Input: part model. Units: mm. Frame: model coordinates. Coordinates: 2 decimals unless noted, no trailing zeros. Write each loop counter-clockwise with the first axis right and the second up, starting at its lowest first coordinate (ties: lowest second). Pieces come first, ordered by that corner, then holes. Notation, with made-up numbers: M -5,48.5 L 36,48.5 A19 cw 36,80.5 Z; hole C 78,78 d11. An arc over 180 degrees is marked long. Write each question's results on one line, items separated by ' | '. Start each with the question number.
1. Ray query, probe 1 along Y at (x, z) = (-6, 5.25); probe 2 along Y at (x, z) = (-11.5, 1); probe 3 along X at (y, z) = (4.5, -4.5). Return the intervals inside material, ascending.
2. Section query A-A, the plane x = -7.5. Output: boundary loops of the cut face in (y, z).
3. First-contact query: pin 1 (8 mm diameter, centred on x = -16, z = -3.5, fed in from +Y); pin 2 (2 mm diameter, centred on x = -9, y = -2.5, fed in from +Z); pin 3 (4 mm diameter, centred on x = -11.5, z = 3, fed in from +Y). Flat tips, straight axial feed; report the tip coordinate or a pass-through.
4. Section query B-B, the plane y = -3.75. Output: boundary loops of the cut face in (x, z).
```python
from build123d import *

# Parameters (mm, degrees)
CROQUIS_BASE_DEPTH             = 6.9937
LENTE_PPAL_1_REACH             = 29.176
LENTE_PPAL_1_DIRECTION_2_REACH = 29.176
LENTE_PPAL_2_DEPTH             = 28.175928622
LENTE_PPAL_2_DEPTH_BACK        = 28.175928622
CROQUIS9_3_OUTSIDE_W           = 30.065
CROQUIS9_3_OUTSIDE_H           = 25.937
LENTE_START                    = -6.9937
LENTE_FRONTAL_DEPTH            = 13.9874
LENTE_START_2                  = -6.993701
LENTE_TRASERA_DEPTH            = 13.987402


with BuildPart() as part:
    # Croquis1 → croquis base (new, symmetric)
    with BuildSketch(Plane.XY):
        with BuildLine():
            Line((-8.981845695, 12.608155172), (-23.035921146, 11.871612288))
            Line((-23.035921146, 11.871612288), (-23.035921146, 11.54013782))
            ThreePointArc((-23.035921146, 11.54013782), (-20.949684518, 9.582335705), (-18.945192114, 7.540918896))
            add(Edge.make_bspline(
                [(-18.945192114, 7.540918896), (-10.215008384, -3.697644103), (-2.846604825, -5.059081104)],
                knots=[0.497667241, 0.497667241, 0.497667241, 0.49955428, 0.49955428, 0.49955428], degree=2, weights=[1, 1, 1]))
            add(Edge.make_bspline(
                [(-2.846604825, -5.059081104), (-2.498165198, -4.87297933), (-2.177330418, -4.684462446)],
                knots=[0.498812075, 0.498812075, 0.498812075, 0.498911556, 0.498911556, 0.498911556], degree=2, weights=[1, 1, 1]))
            Line((-2.177330418, -4.684462446), (-2.177330418, 6.186438919))
            add(Edge.make_bspline(
                [(-2.177330418, 6.186438919), (-4.063319702, 8.141636997), (-6.994875026, 10.477389992)],
                knots=[0.50138293, 0.50138293, 0.50138293, 0.502013312, 0.502013312, 0.502013312], degree=2, weights=[1, 1, 1]))
            Line((-6.994875026, 10.477389992), (-8.981845695, 12.608155172))
        make_face()
    extrude(amount=CROQUIS_BASE_DEPTH, both=True)

    # lente ppal 1: up to this face of the body (flat: up to its plane)
    lente_ppal_1_end = Plane(part.part.faces().sort_by_distance((-10.153546236, 5.159655325, 6.9937))[0])
    # Croquis9 → lente ppal 1 (add, up to the picked face)
    with BuildSketch(Plane.XY, mode=Mode.PRIVATE) as lente_ppal_1_sk1:
        with BuildLine():
            add(Edge.make_bspline(
                [(-2.177330418, -4.388282022), (-10.4130765, -4.994158739), (-19.969359014, 9.493765032)],
                knots=[0, 0, 0, 1, 1, 1], degree=2))
            Line((-19.969359014, 9.493765032), (-10.309820395, 10))
            Line((-10.309820395, 10), (-2.177330418, 6.082860828))
            Line((-2.177330418, 6.082860828), (-2.177330418, 2.424232079))
            add(Edge.make_bspline(
                [(-2.177330418, 2.424232079), (-0.304369248, 0.128042884), (-2.177330418, -1.840420572)],
                knots=[0, 0, 0, 1, 1, 1], degree=2))
            Line((-2.177330418, -1.840420572), (-2.177330418, -4.388282022))
        make_face()
    lente_ppal_1_tool1 = split(extrude(lente_ppal_1_sk1.sketch, amount=LENTE_PPAL_1_REACH, mode=Mode.PRIVATE), bisect_by=lente_ppal_1_end, keep=Keep.BOTH, mode=Mode.PRIVATE)
    add(lente_ppal_1_tool1.solids().sort_by(Axis((-9.106368, 3.599172, 0), (0, 0, 1)))[0])

    # lente ppal 1 direction 2: up to this face of the body (flat: up to its plane)
    lente_ppal_1_direction_2_end = Plane(part.part.faces().sort_by_distance((-10.153546236, 5.159655325, -6.9937))[0])
    # Croquis9 → lente ppal 1 direction 2 (add, up to the picked face)
    with BuildSketch(Plane.XY, mode=Mode.PRIVATE) as lente_ppal_1_direction_2_sk1:
        with BuildLine():
            add(Edge.make_bspline(
                [(-2.177330418, -4.388282022), (-10.4130765, -4.994158739), (-19.969359014, 9.493765032)],
                knots=[0, 0, 0, 1, 1, 1], degree=2))
            Line((-19.969359014, 9.493765032), (-10.309820395, 10))
            Line((-10.309820395, 10), (-2.177330418, 6.082860828))
            Line((-2.177330418, 6.082860828), (-2.177330418, 2.424232079))
            add(Edge.make_bspline(
                [(-2.177330418, 2.424232079), (-0.304369248, 0.128042884), (-2.177330418, -1.840420572)],
                knots=[0, 0, 0, 1, 1, 1], degree=2))
            Line((-2.177330418, -1.840420572), (-2.177330418, -4.388282022))
        make_face()
    lente_ppal_1_direction_2_tool1 = split(extrude(lente_ppal_1_direction_2_sk1.sketch, amount=-LENTE_PPAL_1_DIRECTION_2_REACH, mode=Mode.PRIVATE), bisect_by=lente_ppal_1_direction_2_end, keep=Keep.BOTH, mode=Mode.PRIVATE)
    add(lente_ppal_1_direction_2_tool1.solids().sort_by(Axis((-9.106368, 3.599172, 0), (0, 0, -1)))[0])

    # Croquis9_3 outside → lente ppal 2 (cut, two sides: drawn at the far end of the back side and taken through both)
    with BuildSketch(Plane.XY.offset(-LENTE_PPAL_2_DEPTH_BACK)):
        with Locations((-12.1385, 3.7745)):
            Rectangle(CROQUIS9_3_OUTSIDE_W, CROQUIS9_3_OUTSIDE_H)
        with BuildLine():
            Line((-2.177330418, -1.840420572), (-2.177330418, -4.388282022))
            add(Edge.make_bspline(
                [(-2.177330418, -4.388282022), (-10.4130765, -4.994158739), (-19.969359014, 9.493765032)],
                knots=[0, 0, 0, 1, 1, 1], degree=2))
            Line((-19.969359014, 9.493765032), (-10.309820395, 10))
            Line((-10.309820395, 10), (-2.177330418, 6.082860828))
            Line((-2.177330418, 6.082860828), (-2.177330418, 2.424232079))
            add(Edge.make_bspline(
                [(-2.177330418, 2.424232079), (-0.304369248, 0.128042884), (-2.177330418, -1.840420572)],
                knots=[0, 0, 0, 1, 1, 1], degree=2))
        make_face(mode=Mode.SUBTRACT)
    extrude(amount=LENTE_PPAL_2_DEPTH + LENTE_PPAL_2_DEPTH_BACK, mode=Mode.SUBTRACT)

    # Croquis8 → lente frontal (add)
    with BuildSketch(Plane.XY.offset(LENTE_START)):
        with BuildLine():
            Line((0.1, 2.877673418), (0.1, 15.587903347))
            Line((0.1, 15.587903347), (-1.059110992, 15.277320493))
            Line((-1.059110992, 15.277320493), (-2.200378811, 14.9065001))
            Line((-2.200378811, 14.9065001), (-3.324385438, 14.486251242))
            Line((-3.324385438, 14.486251242), (-4.38392255, 13.922885367))
            Line((-4.38392255, 13.922885367), (-5.329535454, 13.184091597))
            Line((-5.329535454, 13.184091597), (-6.132492182, 12.292317806))
            Line((-6.132492182, 12.292317806), (-6.768395299, 11.274660091))
            Line((-6.768395299, 11.274660091), (-7.217923211, 10.162039465))
            Line((-7.217923211, 10.162039465), (-10.309820395, 10))
            Line((-10.309820395, 10), (-2.177330418, 2.342487007))
            Line((-2.177330418, 2.342487007), (-1.190501641, 2.376947827))
            add(Edge.make_bspline(
                [(-1.190501641, 2.376947827), (-0.463368169, 2.402339888), (0.1, 2.877673418)],
                knots=[0, 0, 0, 1, 1, 1], degree=2))
        make_face()
    extrude(amount=LENTE_FRONTAL_DEPTH)


with BuildPart() as lente_trasera_tool:
    # Croquis11 → lente trasera (new body)
    with BuildSketch(Plane.XY.offset(LENTE_START_2)):
        with BuildLine():
            Line((0.1, -2.367807069), (0.1, -2.867807069))
            Line((0.1, -2.867807069), (-4.723154154, -6))
            Line((-4.723154154, -6), (-9.706405629, -1.513060218))
            Line((-9.706405629, -1.513060218), (-1.458120605, -1.801096678))
            add(Edge.make_bspline(
                [(-1.458120605, -1.801096678), (-0.674591915, -1.828458103), (0.1, -2.367807069)],
                knots=[0, 0, 0, 1, 1, 1], degree=2))
        make_face()
    extrude(amount=LENTE_TRASERA_DEPTH)


with BuildPart() as part_1:
    add(part.part)


with BuildPart() as part_2:
    # lente trasera: joined with lente_trasera_tool
    add(part_1.part.fuse(lente_trasera_tool.part, tol=0.00001))


solid = part_2.part
```
Answer:
1) probe 1: -4.85 to 12.44 | probe 2: -0.6 to 9.94 | probe 3: -16.36 to 0.1
2) outline: M -3.5,-6.99 L 10.15,-6.99 L 10.15,6.99 L -3.5,6.99 Z
3) pin 1: y = 9.91 | pin 2: z = 6.99 | pin 3: y = 10.04
4) outline: M -7.22,-6.99 L -6.37,-6.99 L -1.26,-6.99 L -1.26,6.99 L -6.37,6.99 L -7.22,6.99 Z
